```python
from build123d import *

# Parameters (mm, degrees)
BOSS_EXTRU_1_DEPTH         = 45
BOSS_EXTRU_1_DEPTH_BACK    = 45
CONG_1_R                   = 3
ENL_V_MAT_EXTRU_1_DEPTH    = 2.5
R_P_TITION_LIN_AIRE1_COUNT = 6
R_P_TITION_LIN_AIRE1_PITCH = 5.5
SYM_TRIE1_COPY_1_DEPTH     = 2.5
SYM_TRIE1_COPY_2_DEPTH     = 2.5
SYM_TRIE1_COPY_3_DEPTH     = 2.5
SYM_TRIE1_COPY_4_DEPTH     = 2.5
SYM_TRIE1_COPY_5_DEPTH     = 2.5


with BuildPart() as part:
    # Esquisse1 → Boss.-Extru.1 (new, two sides: drawn at the far end of the back side and taken through both)
    with BuildSketch(Plane(origin=(0, 0, 0), x_dir=(0, 0, -1), z_dir=(1, 0, 0)).offset(-BOSS_EXTRU_1_DEPTH_BACK)):
        Polygon((-48.25, 40), (0, 40), (0, 0), (0, -40), (-24, -40), (-48.25, -25), align=None)
    extrude(amount=BOSS_EXTRU_1_DEPTH + BOSS_EXTRU_1_DEPTH_BACK)

    # Cong_1
    cong_1_edges = [part.edges().sort_by_distance(p)[0] for p in [
        (0, -40, 0),
        (0, -40, 24),
        (0, -25, 48.25),
        (0, 40, 48.25),
        (0, 40, 0),
    ]]
    fillet(cong_1_edges, radius=CONG_1_R)

    # Esquisse2 → Enl_v. mat.-Extru.1 (cut)
    with BuildSketch(Plane(origin=(45, 0, 0), x_dir=(0, 0, -1), z_dir=(1, 0, 0))):
        with BuildLine():
            Line((-40.074077662, 21.746799664), (-8.626027221, 21.746799664))
            ThreePointArc((-8.626027221, 21.746799664), (-7.226027221, 20.346799664), (-8.626027221, 18.946799664))
            Line((-8.626027221, 18.946799664), (-40.074077662, 18.946799664))
            ThreePointArc((-40.074077662, 18.946799664), (-41.474077662, 20.346799664), (-40.074077662, 21.746799664))
        make_face()
    enl_v_mat_extru_1 = extrude(amount=-ENL_V_MAT_EXTRU_1_DEPTH, mode=Mode.SUBTRACT)

    # R_p_tition lin_aire1: Enl_v. mat.-Extru.1 ×6
    with Locations(*[(0, -i * R_P_TITION_LIN_AIRE1_PITCH, 0) for i in range(1, R_P_TITION_LIN_AIRE1_COUNT)]):
        add(enl_v_mat_extru_1, mode=Mode.SUBTRACT)

    # Sym_trie1: Enl_v. mat.-Extru.1 across plane
    add(enl_v_mat_extru_1.mirror(Plane(origin=(0, 0, 0), x_dir=(0, 0, 1), z_dir=(1, 0, 0))), mode=Mode.SUBTRACT)

    # Sym_trie1 copy 1 sketch → Sym_trie1 copy 1 (cut)
    with BuildSketch(Plane(origin=(-45, -5.5, 0), x_dir=(0, 0, -1), z_dir=(-1, 0, 0))):
        with BuildLine():
            Line((-40.074077662, -21.746799664), (-8.626027221, -21.746799664))
            ThreePointArc((-8.626027221, -21.746799664), (-7.226027221, -20.346799664), (-8.626027221, -18.946799664))
            Line((-8.626027221, -18.946799664), (-40.074077662, -18.946799664))
            ThreePointArc((-40.074077662, -18.946799664), (-41.474077662, -20.346799664), (-40.074077662, -21.746799664))
        make_face()
    extrude(amount=-SYM_TRIE1_COPY_1_DEPTH, mode=Mode.SUBTRACT)

    # Sym_trie1 copy 2 sketch → Sym_trie1 copy 2 (cut)
    with BuildSketch(Plane(origin=(-45, -11, 0), x_dir=(0, 0, -1), z_dir=(-1, 0, 0))):
        with BuildLine():
            Line((-40.074077662, -21.746799664), (-8.626027221, -21.746799664))
            ThreePointArc((-8.626027221, -21.746799664), (-7.226027221, -20.346799664), (-8.626027221, -18.946799664))
            Line((-8.626027221, -18.946799664), (-40.074077662, -18.946799664))
            ThreePointArc((-40.074077662, -18.946799664), (-41.474077662, -20.346799664), (-40.074077662, -21.746799664))
        make_face()
    extrude(amount=-SYM_TRIE1_COPY_2_DEPTH, mode=Mode.SUBTRACT)

    # Sym_trie1 copy 3 sketch → Sym_trie1 copy 3 (cut)
    with BuildSketch(Plane(origin=(-45, -16.5, 0), x_dir=(0, 0, -1), z_dir=(-1, 0, 0))):
        with BuildLine():
            Line((-40.074077662, -21.746799664), (-8.626027221, -21.746799664))
            ThreePointArc((-8.626027221, -21.746799664), (-7.226027221, -20.346799664), (-8.626027221, -18.946799664))
            Line((-8.626027221, -18.946799664), (-40.074077662, -18.946799664))
            ThreePointArc((-40.074077662, -18.946799664), (-41.474077662, -20.346799664), (-40.074077662, -21.746799664))
        make_face()
    extrude(amount=-SYM_TRIE1_COPY_3_DEPTH, mode=Mode.SUBTRACT)

    # Sym_trie1 copy 4 sketch → Sym_trie1 copy 4 (cut)
    with BuildSketch(Plane(origin=(-45, -22, 0), x_dir=(0, 0, -1), z_dir=(-1, 0, 0))):
        with BuildLine():
            Line((-40.074077662, -21.746799664), (-8.626027221, -21.746799664))
            ThreePointArc((-8.626027221, -21.746799664), (-7.226027221, -20.346799664), (-8.626027221, -18.946799664))
            Line((-8.626027221, -18.946799664), (-40.074077662, -18.946799664))
            ThreePointArc((-40.074077662, -18.946799664), (-41.474077662, -20.346799664), (-40.074077662, -21.746799664))
        make_face()
    extrude(amount=-SYM_TRIE1_COPY_4_DEPTH, mode=Mode.SUBTRACT)

    # Sym_trie1 copy 5 sketch → Sym_trie1 copy 5 (cut)
    with BuildSketch(Plane(origin=(-45, -27.5, 0), x_dir=(0, 0, -1), z_dir=(-1, 0, 0))):
        with BuildLine():
            Line((-40.074077662, -21.746799664), (-8.626027221, -21.746799664))
            ThreePointArc((-8.626027221, -21.746799664), (-7.226027221, -20.346799664), (-8.626027221, -18.946799664))
            Line((-8.626027221, -18.946799664), (-40.074077662, -18.946799664))
            ThreePointArc((-40.074077662, -18.946799664), (-41.474077662, -20.346799664), (-40.074077662, -21.746799664))
        make_face()
    extrude(amount=-SYM_TRIE1_COPY_5_DEPTH, mode=Mode.SUBTRACT)


solid = part.part
```
Source: CAD feature listing. Evaluate the final solid. Frame: model axes, mm. A direction names the side the tool comes from. Coordinates: 2 decimals unless noted, no trailing zeros. Write each loop counter-clockwise with the first axis right and the second up, starting at its lowest first coordinate (ties: lowest second). Pieces come first, ordered by that corner, then holes. Notation, with made-up numbers: M 64,39.5 L 85,39.5 A33 ccw 85,74.5 Z; hole C 40,-25.5 d4. An arc over 180 degrees is marked long. Answer as a JSON object with one key per item and string values.
1. Cut plane D-D on y = -34. Output: boundary loops of the cut face in (x, z), plus the area to 3 significant figures.
Evaluation:
{"outline": "M -45,0 L 45,0 L 45,33.7 L -45,33.7 Z", "area": "3,030 mm^2"}
2. Cut plane A-A on x = -31.5. Output: boundary loops of the cut face in (y, z).
Evaluation:
{"outline": "M -40,3 A3 ccw -37,0 L 37,0 A3 ccw 40,3 L 40,45.25 A3 ccw 37,48.25 L -23.33,48.25 A3 ccw -25.88,46.83 L -39.55,24.73 A3 ccw -40,23.15 Z"}
3. Access query for faces 4 (the flat face through (-42.5, 9, 25)), 5 (the cylindrical face through (0.63, 39.14, 47.35)), 6 (the cylindrical face through (43.768, -7.122, 7.226)). Directions: +Z, -Z, +X, -X, +Y, -Y. A direction counts if a zero-diameter tool reaches every point of the face in a straight line with its end or side. Return the directions, or none.
Evaluation:
{"face 4": "-X", "face 5": "+Z, +X, -X, +Y", "face 6": "+X"}
4. Cut plane B-B on y = -2. Output: boundary loops of the cut face in (x, z), plus the area to 3 significant figures.
Evaluation:
{"outline": "M -45,0 L 45,0 L 45,7.27 L 42.5,7.27 L 42.5,41.43 L 45,41.43 L 45,48.25 L -45,48.25 L -45,41.43 L -42.5,41.43 L -42.5,7.27 L -45,7.27 Z", "area": "4,170 mm^2"}
5. Draft query along Y for faces 1 (the cylindrical face through (0.63, -39.1, 0.86)), 2 (the flat face through (-44, -5.753, 25)), 3 (the cylindrical face through (0.63, 39.14, 0.9)). Return one class per face: released by +Y, released by -Y, zero draft, split by the parting line, or undercut.
Evaluation:
{"face 1": "released by -Y", "face 2": "undercut", "face 3": "released by +Y"}
6. Cut plane C-C on z = 43.5. Output: boundary loops of the cut face in (x, y), plus the area to 3 significant figures.
Evaluation:
{"outline": "M -45,-27.94 L 45,-27.94 L 45,40 L -45,40 Z", "area": "6,110 mm^2"}
7. Ray query, L1, parallel to X at y = -1, z = 18; L2, parallel to Z at x = -23, y = -27; L3, parallel to Y at x = 5, z = 38. Return the intervals inside material, ascending.
Evaluation:
{"L1": "-42.5 to 42.5", "L2": "0 to 45.02", "L3": "-31.34 to 40"}
8. Contact query for flat-ended pins moving along their axis: P1, Ø3, axis at x = -43, z = 30.5, coming from the -Y side; P2, Ø1.4, axis at y = 21, z = 21.5, coming from the -X side; P3, Ø3, axis at x = 44.5, z = 25.5, coming from the -Y side; P4, Ø1, axis at y = -29, z = 43, coming from the -X side. Output: stop coordinate, or through.
Evaluation:
{"P1": "y = -36.91", "P2": "x = -42.5", "P3": "y = -39.88", "P4": "through"}
